from build123d import *

# Parameters (mm, degrees)
BOSS_EXTRUDE2_DEPTH = 40
SKETCH3_W           = 63.5
SKETCH3_H           = 50.713358162
BOSS_EXTRUDE3_DEPTH = 5
SKETCH5_W           = 40
SKETCH5_H           = 26.795354342
BOSS_EXTRUDE4_DEPTH = 45
SKETCH7_R           = 25
BOSS_EXTRUDE6_DEPTH = 2
SKETCH11_R          = 6
BOSS_EXTRUDE7_DEPTH = 6
SKETCH13_R          = 3.25
BOSS_EXTRUDE8_DEPTH = 25


with BuildPart() as part:
    # Sketch1 → Boss-Extrude2 (new body)
    with BuildSketch(Plane.XY):
        with BuildLine():
            ThreePointArc((5.08, 33.118635635), (0, 52.077453737), (-5.08, 33.118635635))
            Line((-5.08, 33.118635635), (-21.263810414, 5.087453737))
            Line((-21.263810414, 5.087453737), (-26.343810414, 5.087453737))
            Line((-26.343810414, 5.087453737), (-26.343810414, 6.865453737))
            Line((-26.343810414, 6.865453737), (-31.75, 6.865453737))
            Line((-31.75, 6.865453737), (-31.75, 57.578811899))
            Line((-31.75, 57.578811899), (31.75, 57.578811899))
            Line((31.75, 57.578811899), (31.75, 6.865453737))
            Line((31.75, 6.865453737), (26.343810414, 6.865453737))
            Line((26.343810414, 6.865453737), (26.343810414, 5.087453737))
            Line((26.343810414, 5.087453737), (21.263810414, 5.087453737))
            Line((21.263810414, 5.087453737), (5.08, 33.118635635))
        make_face()
    extrude(amount=BOSS_EXTRUDE2_DEPTH)

    # Sketch3 → Boss-Extrude3 (add)
    with BuildSketch(Plane.XY.offset(40)):
        with Locations((0, 32.222132818)):
            Rectangle(SKETCH3_W, SKETCH3_H)
    extrude(amount=BOSS_EXTRUDE3_DEPTH)

    # Sketch5 → Boss-Extrude4 (add)
    with BuildSketch(Plane.XY.offset(45)):
        with Locations((-51.75, 31.186442922)):
            Rectangle(SKETCH5_W, SKETCH5_H)
    extrude(amount=-BOSS_EXTRUDE4_DEPTH)

    # Sketch7 → Boss-Extrude6 (add)
    with BuildSketch(Plane.XZ.offset(-17.788765751)):
        with Locations((-71.75, 22.5)):
            Circle(SKETCH7_R)
    extrude(amount=-BOSS_EXTRUDE6_DEPTH)

    # Sketch11 → Boss-Extrude7 (add)
    with BuildSketch(Plane(origin=(0, 17.788765751, 0), x_dir=(-1, 0, 0), z_dir=(0, -1, 0))):
        with Locations(Location((84.7850913, -22.5, 0), (0, 0, 90))):
            Circle(SKETCH11_R)
    extrude(amount=-BOSS_EXTRUDE7_DEPTH)

    # Sketch13 → Boss-Extrude8 (add)
    with BuildSketch(Plane(origin=(0, 23.788765751, 0), x_dir=(1, 0, 0), z_dir=(0, 1, 0))):
        with Locations(Location((-84.7850913, -22.5, 0), (0, 0, 270))):
            Circle(SKETCH13_R)
    extrude(amount=BOSS_EXTRUDE8_DEPTH)


solid = part.part
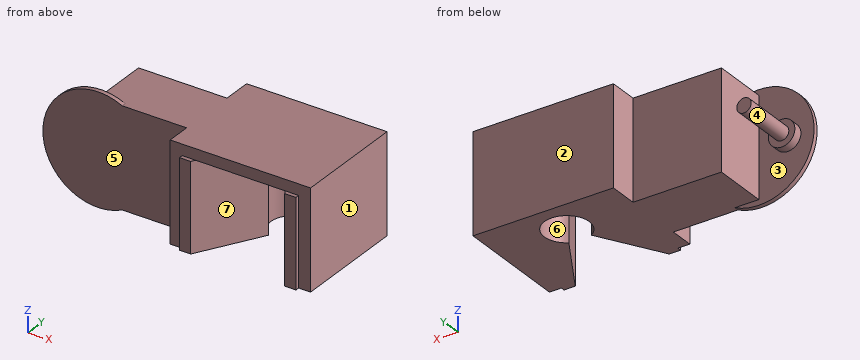
The listing builds one solid part. Answer for the finished solid, in the listing's coordinates (mm). Face numbers are marked on the shaded views. A direction names the side the tool comes from. Give positions to 0.01 mm unless a question says otherwise; leave off trailing zeros. Loops run counter-clockwise (first coordinate to the right, second up) from the corner with the lowest first, then second, coordinate; pieces in that order, holes last. Notation, with made-up numbers: (8, -9.75) - (51, -9.75) arc R19 ccw to (51, 18.25) - close; hole circle Ø6 at (68.25, 29.5). An arc over 180 degrees is marked (long way). Write each question's results on one line, items separated by ' | '.
1. Find section B-B, the plane z = 22.5. Write down the section's boundary in (x, y).
Resolved:
outline: (-96.75, 17.79) - (-31.75, 17.79) - (-31.75, 6.87) - (-26.34, 6.87) - (-26.34, 5.09) - (-21.26, 5.09) - (-5.08, 33.12) arc R10.16 cw (long way) to (5.08, 33.12) - (21.26, 5.09) - (26.34, 5.09) - (26.34, 6.87) - (31.75, 6.87) - (31.75, 57.58) - (-31.75, 57.58) - (-31.75, 44.58) - (-71.75, 44.58) - (-71.75, 19.79) - (-78.79, 19.79) - (-78.79, 23.79) - (-81.54, 23.79) - (-81.54, 48.79) - (-88.04, 48.79) - (-88.04, 23.79) - (-90.79, 23.79) - (-90.79, 19.79) - (-96.75, 19.79) - close
2. Flat-ended cylindrical pins translate along their axes: P1, Ø3.5, axis at x = -87.5, z = 25.5, coming from the +Y side; P2, Ø8.5, axis at y = 13, z = 31.5, coming from the -X side; P3, Ø6, axis at x = -69, z = 11.5, coming from the +Y side. Find the tip coordinate at first contact, or state that the pin passes through.
Resolved:
P1: stops at y = 48.79 | P2: stops at x = -31.75 | P3: stops at y = 44.58
3. Find section A-A, the plane y = 22.5. Write down the section's boundary in (x, z).
Resolved:
outline: circle Ø12 at (-84.79, 22.5); (-71.75, 0) - (-11.21, 0) - (-11.21, 40) - (11.21, 40) - (11.21, 0) - (31.75, 0) - (31.75, 45) - (-71.75, 45) - close
4. For a pull along X with two mould halves and no side action, classify the marked faces 1, 2 and 3 as +X half, -X half, draft (parallel to the pull), parting line (faces both ways), or undercut.
Resolved:
face 1: +X half | face 2: draft | face 3: undercut
5. Find section D-D, the plane y = 50.5. Write down the section's boundary in (x, z).
Resolved:
outline: (-31.75, 0) - (-5.44, 0) - (-5.44, 40) - (5.44, 40) - (5.44, 0) - (31.75, 0) - (31.75, 45) - (-31.75, 45) - close
6. Which of the six approach directions +Z, -Z, +X, -X, +Y, -Y give full straight-line access (tool end or side, diameter ignored) to the marked faces 4, 5, 6 and 7?
Resolved:
face 4: +Y | face 5: +Z, -Z, -X, -Y | face 6: -Z | face 7: -Z, -Y
7. Consider probe 1 along X at (y, z) = (28.5, 24.5); probe 2 along X at (y, z) = (42, 19); probe 3 along Z at (x, y) = (-71, 39.5). Determine where each line is inside the solid, lowest interval first. Write a range as from..to.
Resolved:
probe 1: x = -87.35..-82.22, -71.75..-7.75, 7.75..31.75 | probe 2: x = -71.75..-10.16, 10.16..31.75 | probe 3: z = 0..45
8. Find section C-C, the plane x = 0. Write down the section's boundary in (y, z), then the cut area to 3 significant figures.
Resolved:
outline: (6.87, 40) - (52.08, 40) - (52.08, 0) - (57.58, 0) - (57.58, 45) - (6.87, 45) - close | area: 474 mm^2
